```python
from build123d import *

# Parameters (mm, degrees)
BOSS_EXTRUDE1_DEPTH       = 70
FILLET1_R                 = 5
FILLET2_R                 = 5
M4X0_7_TAPPED_HOLE1_D     = 3.3
M4X0_7_TAPPED_HOLE1_DEPTH = 5
SKETCH13_R                = 25
CUT_EXTRUDE1_DEPTH        = 4
SKETCH14_R                = 17.9
CUT_EXTRUDE2_DEPTH        = 2
SKETCH15_R                = 17.5
CUT_EXTRUDE3_DEPTH        = 4
SKETCH16_R                = 13
CUT_EXTRUDE4_DEPTH        = 84.815273071
SKETCH17_R                = 17.9
CUT_EXTRUDE5_DEPTH        = 3


with BuildPart() as part:
    # Sketch1 → Boss-Extrude1 (new body)
    with BuildSketch(Plane.XY):
        Polygon((0, -30), (0, -35), (34, -35), (34, 35), (0, 35), (0, 30), (20, 30), (20, -30), align=None)
    extrude(amount=BOSS_EXTRUDE1_DEPTH)

    # Fillet1
    fillet1_edges = [part.edges().sort_by_distance(p)[0] for p in [
        (17, -35, 70),
        (17, -35, 0),
        (17, 35, 0),
        (17, 35, 70),
    ]]
    fillet(fillet1_edges, radius=FILLET1_R - 0.0001)  # a hair under: the kernel refuses the full size

    # Fillet2
    fillet2_edges = [part.edges().sort_by_distance(p)[0] for p in [
        (34, 0, 70),
        (34, 0, 0),
        (34, 35, 35),
        (34, -35, 35),
        (34, 33.535563195, 68.535563195),
        (34, 33.535563195, 1.464436805),
        (34, -33.535563195, 1.464436805),
        (34, -33.535563195, 68.535563195),
    ]]
    fillet(fillet2_edges, radius=FILLET2_R - 0.0001)  # a hair under: the kernel refuses the full size

    # M4x0.7 Tapped Hole1
    with Locations(Plane(origin=(0, 35, 0), x_dir=(1, 0, 0), z_dir=(0, 1, 0))):
        with Locations((10, -12.5), (10, -27.5), (10, -42.5), (10, -57.5)):
            m4x0_7_tapped_hole1 = Hole(M4X0_7_TAPPED_HOLE1_D / 2, depth=M4X0_7_TAPPED_HOLE1_DEPTH)

    # Mirror1: M4x0.7 Tapped Hole1 across plane
    add(m4x0_7_tapped_hole1.mirror(Plane.ZX), mode=Mode.SUBTRACT)

    # Sketch13 → Cut-Extrude1 (cut)
    with BuildSketch(Plane.ZY.offset(-20)):
        with Locations((35, 0)):
            Circle(SKETCH13_R)
    extrude(amount=-CUT_EXTRUDE1_DEPTH, mode=Mode.SUBTRACT)

    # Sketch14 → Cut-Extrude2 (cut)
    with BuildSketch(Plane.ZY.offset(-24)):
        with Locations((35, 0)):
            Circle(SKETCH14_R)
    extrude(amount=-CUT_EXTRUDE2_DEPTH, mode=Mode.SUBTRACT)

    # Sketch15 → Cut-Extrude3 (cut)
    with BuildSketch(Plane.ZY.offset(-26)):
        with Locations((35, 0)):
            Circle(SKETCH15_R)
    extrude(amount=-CUT_EXTRUDE3_DEPTH, mode=Mode.SUBTRACT)

    # Sketch16 → Cut-Extrude4 (cut, through all)
    with BuildSketch(Plane.ZY.offset(-30)):
        with Locations((35, 0)):
            Circle(SKETCH16_R)
    extrude(amount=-CUT_EXTRUDE4_DEPTH, mode=Mode.SUBTRACT)

    # Sketch17 → Cut-Extrude5 (cut)
    with BuildSketch(Plane.ZY.offset(-26)):
        with Locations((35, 0)):
            Circle(SKETCH17_R)
    extrude(amount=-CUT_EXTRUDE5_DEPTH, mode=Mode.SUBTRACT)


solid = part.part
```
Build history of the part. All positions in model axes, mm. A direction names the side the tool comes from. Coordinates: 2 decimals unless noted, no trailing zeros. Order: outer loops, then holes, each group sorted by start corner. A loop starts at its lowest first (then second) coordinate and runs counter-clockwise, first axis right, second up. Notation, with made-up numbers: (32.25, 19) -> (41.25, 19) arc R20 cw to (41.25, 25) -> close; hole circle Ø9 at (58.25, 3). An arc over 180 degrees is marked (long way). Answer in a Markdown table with one row per item. Add a question column.
Q1. Which spindle directions (+Z, -Z, +X, -X, +Y, -Y) get a long thin tool onto all of the face, cutting with end or side? Do faces 4 (the face through (0, -32, 35)), 5 (the face through (10, 30, 35)), 6 (the face through (24, -11, 51)). Say none if no direction does.
Q2. Drop a flat-ended pin along its axis: pin 1 (15 mm diameter, centred on y = 6.5, z = 39, fed in from -X). Give the stop position or say it passes through.
Q3. Band-saw the part on D-D, the plane z = 42.5. Give the number of separate pieces and of enclosed holes in the cut face, then the cut area to 3 significant figures.
Q4. Band-saw the part on B-B, the plane y = 0. List the corners of the cut face in (x, z).
Q5. Wall check: line 1 along Y through (x, z) = (13.5, 17); line 2 along Z through (x, y) = (10, 31.5); line 3 along X through (y, z) = (13.5, 24.5). Give the ranges that are in metal, low to high. Write a range as [from, to].
Q6. Band-saw the part on C-C, the plane z = 57.5. List the corners of the cut face in (x, y).
Q7. Mould opens along Z. For faces 1 (the face through (9.239, 32.465, 13.964)), 2 (the face through (24, 0, 70)), 3 (the face through (32, -34, 35)) say: +Z half, -Z half, draft (parallel to the pull), parting line (faces both ways), or undercut.
Answers follow:
| question | item | result |
|---|---|---|
| 1 | face 4 | +Z, -Z, -X, +Y, -Y |
| 1 | face 5 | +Z, -Z, -X |
| 1 | face 6 | -X |
| 2 | pin 1 | x = 30 |
| 3 | separate pieces | 4 |
| 3 | enclosed holes | 0 |
| 3 | area | 666 mm^2 |
| 4 | outline | (20, 0) -> (29, 0) arc R5 ccw to (34, 5) -> (34, 22) -> (30, 22) -> (30, 17.5) -> (29, 17.5) -> (29, 17.1) -> (24, 17.1) -> (24, 10) -> (20, 10) -> close; (20, 60) -> (24, 60) -> (24, 52.9) -> (29, 52.9) -> (29, 52.5) -> (30, 52.5) -> (30, 48) -> (34, 48) -> (34, 65) arc R5 ccw to (29, 70) -> (20, 70) -> close |
| 5 | line 1 | [-35, -30], [30, 35] |
| 5 | line 2 | [0.23, 10.85], [14.15, 25.85], [29.15, 40.85], [44.15, 55.85], [59.15, 69.77] |
| 5 | line 3 | [30, 34] |
| 6 | outline | (0, -35) -> (8.35, -35) -> (8.35, -30) -> (0, -30) -> close; (0, 30) -> (8.35, 30) -> (8.35, 35) -> (0, 35) -> close; (11.65, -35) -> (29, -35) arc R5 ccw to (34, -30) -> (34, 30) arc R5 ccw to (29, 35) -> (11.65, 35) -> (11.65, 30) -> (20, 30) -> (20, 10.9) -> (24, 10.9) -> (24, -10.9) -> (20, -10.9) -> (20, -30) -> (11.65, -30) -> close |
| 7 | face 1 | undercut |
| 7 | face 2 | +Z half |
| 7 | face 3 | draft |
